from build123d import *

# Parameters (mm, degrees)
BOSS_EXTRUDE1_DEPTH = 1.5
BOSS_EXTRUDE2_DEPTH = 5
SKETCH3_W           = 25
SKETCH3_H           = 17
BOSS_EXTRUDE3_DEPTH = 3


with BuildPart() as part:
    # Sketch1 → Boss-Extrude1 (new body)
    with BuildSketch(Plane(origin=(0, 0, 0), x_dir=(1, 0, 0), z_dir=(0, 1, 0))):
        Polygon((0, 30), (0, 0), (7.5, 0), (7.5, 3), (22.5, 3), (22.5, 0), (30, 0), (30, 30), align=None)
    extrude(amount=BOSS_EXTRUDE1_DEPTH)

    # Sketch2 → Boss-Extrude2 (add)
    with BuildSketch(Plane(origin=(0, 1.5, 0), x_dir=(1, 0, 0), z_dir=(0, 1, 0))):
        Polygon((25, 5.5), (27.5, 5.5), (27.5, 27.5), (2.5, 27.5), (2.5, 5.5), (5, 5.5), align=None)
    extrude(amount=BOSS_EXTRUDE2_DEPTH)

    # Sketch3 → Boss-Extrude3 (add)
    with BuildSketch(Plane.XZ):
        with Locations((15, -19)):
            Rectangle(SKETCH3_W, SKETCH3_H)
    extrude(amount=BOSS_EXTRUDE3_DEPTH)


solid = part.part
Model file for the job. Use its own axes, mm. A direction names the side the tool comes from. Give positions to 0.01 mm unless a question says otherwise; leave off trailing zeros. Loops run counter-clockwise (first coordinate to the right, second up) from the corner with the lowest first, then second, coordinate; pieces in that order, holes last.
1) Tool access for faces 1 (the flat face through (2.5, 4, -17)), 2 (the flat face through (15, -1, -10.5)), 3 (the flat face through (27.5, 4, -16)): list every direction of +Z, -Z, +X, -X, +Y, -Y with a clear straight run to the whole face (end or side of a thin tool).
2) Pull direction X, two halves, no side cores. Call faces 4 (the flat face through (27.5, -1, -19)), 5 (the flat face through (15, 1, -3)), 6 (the flat face through (15, 1, -30)), 7 (the flat face through (22.5, 1, -2)): +X half, -X half, draft (parallel to the pull), parting line (faces both ways), or undercut.
3) Saw through at B-B (z = -15). Write the cut outline in (x, y), plus the area to 3 significant figures.
4) Saw through at C-C (y = 4.25). Write the cut outline in (x, z).
5) Wall check: line 1 (X direction, y = 6.25, z = -21.75); line 2 (Y direction, x = 8.75, z = -10); line 3 (Y direction, x = 27.75, z = -18). Give the ranges that are in metal, low to high.
6) Saw through at D-D (z = -8). Write the cut outline in (x, y), plus the area to 3 significant figures.
7) Saw through at A-A (x = 8.75). Write the cut outline in (y, z).
8) Flat gauge pins, fed straight in: pin 1 Ø3 at (x, y) = (20.5, 4.5) entering from -Z; pin 2 Ø1.5 at (y, z) = (4, -20.5) entering from +X; pin 3 Ø0.9 at (x, y) = (20, -2) entering from +Z. Where does each tip first touch, or does it go through?
Answer block:
1. face 1: +Z, -Z, -X, +Y
1. face 2: +Z, +X, -X, -Y
1. face 3: +Z, -Z, +X, +Y
2. face 4: +X half
2. face 5: undercut
2. face 6: draft
2. face 7: undercut
3. outline: (0, 0) - (2.5, 0) - (2.5, -3) - (27.5, -3) - (27.5, 0) - (30, 0) - (30, 1.5) - (27.5, 1.5) - (27.5, 6.5) - (2.5, 6.5) - (2.5, 1.5) - (0, 1.5) - close
3. area: 245 mm2
4. outline: (2.5, -27.5) - (27.5, -27.5) - (27.5, -5.5) - (2.5, -5.5) - close
5. line 1: x = 2.5 to 27.5
5. line 2: y = 0 to 6.5
5. line 3: y = 0 to 1.5
6. outline: (0, 0) - (30, 0) - (30, 1.5) - (27.5, 1.5) - (27.5, 6.5) - (2.5, 6.5) - (2.5, 1.5) - (0, 1.5) - close
6. area: 170 mm2
7. outline: (-3, -27.5) - (0, -27.5) - (0, -30) - (1.5, -30) - (1.5, -27.5) - (6.5, -27.5) - (6.5, -5.5) - (1.5, -5.5) - (1.5, -3) - (0, -3) - (0, -10.5) - (-3, -10.5) - close
8. pin 1: stops at z = -27.5
8. pin 2: stops at x = 27.5
8. pin 3: stops at z = -10.5
